Model file for the job. Use its own axes, mm. Give positions to 0.01 mm unless a question says otherwise; leave off trailing zeros. Order: outer loops, then holes, each group sorted by start corner. A loop starts at its lowest first (then second) coordinate and runs counter-clockwise, first axis right, second up. Notation, with made-up numbers: (6, 9) - (51, 9) arc R21 cw to (51, 14) - close; hole circle Ø11 at (8, 67). An arc over 180 degrees is marked (long way). Return JSON: item names as keys, results as strings. Group by question number.
from build123d import *

# Parameters (mm, degrees)
SKETCH1_W               = 180
SKETCH1_H               = 95
BOSS_EXTRUDE1_DEPTH     = 3.18
SKETCH2_W               = 3.18
SKETCH2_H               = 37.625
CUT_EXTRUDE1_DEPTH      = 1
CUT_EXTRUDE1_DEPTH_BACK = 4.18
SKETCH3_R               = 1.55
CUT_EXTRUDE2_DEPTH      = 1
CUT_EXTRUDE2_DEPTH_BACK = 4.18
CUT_EXTRUDE3_DEPTH      = 1
CUT_EXTRUDE3_DEPTH_BACK = 4.18
CUT_EXTRUDE4_DEPTH      = 1
CUT_EXTRUDE4_DEPTH_BACK = 4.18
CUT_EXTRUDE5_DEPTH      = 1
CUT_EXTRUDE5_DEPTH_BACK = 4.18
SKETCH8_W               = 58.994769075
SKETCH8_H               = 13
CUT_EXTRUDE6_DEPTH      = 1
CUT_EXTRUDE6_DEPTH_BACK = 4.18
SKETCH9_R               = 1.6
CUT_EXTRUDE7_DEPTH      = 1
CUT_EXTRUDE7_DEPTH_BACK = 4.18


with BuildPart() as part:
    # Sketch1 → Boss-Extrude1 (new body)
    with BuildSketch(Plane.XY):
        Rectangle(SKETCH1_W, SKETCH1_H)
    extrude(amount=BOSS_EXTRUDE1_DEPTH)

    # Sketch2 → Cut-Extrude1 (cut, two sides)
    with BuildSketch(Plane.XY.offset(3.18)) as cut_extrude1_sk:
        with Locations((88.41, 28.6875)):
            Rectangle(SKETCH2_W, SKETCH2_H)
        with Locations((88.41, -28.6875)):
            Rectangle(SKETCH2_W, SKETCH2_H)
    extrude(amount=CUT_EXTRUDE1_DEPTH, mode=Mode.SUBTRACT)
    extrude(cut_extrude1_sk.sketch, amount=-CUT_EXTRUDE1_DEPTH_BACK, mode=Mode.SUBTRACT)

    # Sketch3 → Cut-Extrude2 (cut, two sides)
    with BuildSketch(Plane.XY.offset(3.18)) as cut_extrude2_sk:
        with Locations((88, 0)):
            Circle(SKETCH3_R)
    extrude(amount=CUT_EXTRUDE2_DEPTH, mode=Mode.SUBTRACT)
    extrude(cut_extrude2_sk.sketch, amount=-CUT_EXTRUDE2_DEPTH_BACK, mode=Mode.SUBTRACT)

    # Sketch5 → Cut-Extrude3 (cut, two sides)
    with BuildSketch(Plane(origin=(0, 0, 0), x_dir=(-1, 0, 0), z_dir=(0, 0, -1))) as cut_extrude3_sk:
        Polygon((11.59, 47.5), (-8.41, 47.5), (-8.41, 44.32), (0.09, 44.32), (0.09, 40.32), (-1.91, 40.32), (-1.91, 37.5), (0.09, 37.5), (0.09, 34.5), (3.09, 34.5), (3.09, 37.5), (5.09, 37.5), (5.09, 40.32), (3.09, 40.32), (3.09, 44.32), (11.59, 44.32), align=None)
    extrude(amount=CUT_EXTRUDE3_DEPTH, mode=Mode.SUBTRACT)
    extrude(cut_extrude3_sk.sketch, amount=-CUT_EXTRUDE3_DEPTH_BACK, mode=Mode.SUBTRACT)

    # Sketch6 → Cut-Extrude4 (cut, two sides)
    with BuildSketch(Plane.XY.offset(3.18)) as cut_extrude4_sk:
        Polygon((-21.59, -47.5), (-1.59, -47.5), (-1.59, -44.32), (-10.09, -44.32), (-10.09, -40.32), (-8.09, -40.32), (-8.09, -37.5), (-10.09, -37.5), (-10.09, -34.5), (-13.09, -34.5), (-13.09, -37.5), (-15.09, -37.5), (-15.09, -40.32), (-13.09, -40.32), (-13.09, -44.32), (-21.59, -44.32), align=None)
    extrude(amount=CUT_EXTRUDE4_DEPTH, mode=Mode.SUBTRACT)
    extrude(cut_extrude4_sk.sketch, amount=-CUT_EXTRUDE4_DEPTH_BACK, mode=Mode.SUBTRACT)

    # Sketch7 → Cut-Extrude5 (cut, two sides)
    with BuildSketch(Plane.XY.offset(3.18)) as cut_extrude5_sk:
        Polygon((-90, 10), (-86.82, 10), (-86.82, 1.5), (-82.82, 1.5), (-82.82, 3.5), (-80, 3.5), (-80, 1.5), (-77, 1.5), (-77, -1.5), (-80, -1.5), (-80, -3.5), (-82.82, -3.5), (-82.82, -1.5), (-86.82, -1.5), (-86.82, -10), (-90, -10), align=None)
    extrude(amount=CUT_EXTRUDE5_DEPTH, mode=Mode.SUBTRACT)
    extrude(cut_extrude5_sk.sketch, amount=-CUT_EXTRUDE5_DEPTH_BACK, mode=Mode.SUBTRACT)

    # Sketch8 → Cut-Extrude6 (cut, two sides)
    with BuildSketch(Plane.XY.offset(3.18)) as cut_extrude6_sk:
        with Locations((-57.357372864, -23.3)):
            Rectangle(SKETCH8_W, SKETCH8_H)
    extrude(amount=CUT_EXTRUDE6_DEPTH, mode=Mode.SUBTRACT)
    extrude(cut_extrude6_sk.sketch, amount=-CUT_EXTRUDE6_DEPTH_BACK, mode=Mode.SUBTRACT)

    # Sketch9 → Cut-Extrude7 (cut, two sides)
    with BuildSketch(Plane.XY.offset(3.18)) as cut_extrude7_sk:
        with Locations((-4.59, -27.32)):
            Circle(SKETCH9_R)
        with Locations((43.41, -27.32)):
            Circle(SKETCH9_R)
    extrude(amount=CUT_EXTRUDE7_DEPTH, mode=Mode.SUBTRACT)
    extrude(cut_extrude7_sk.sketch, amount=-CUT_EXTRUDE7_DEPTH_BACK, mode=Mode.SUBTRACT)


solid = part.part
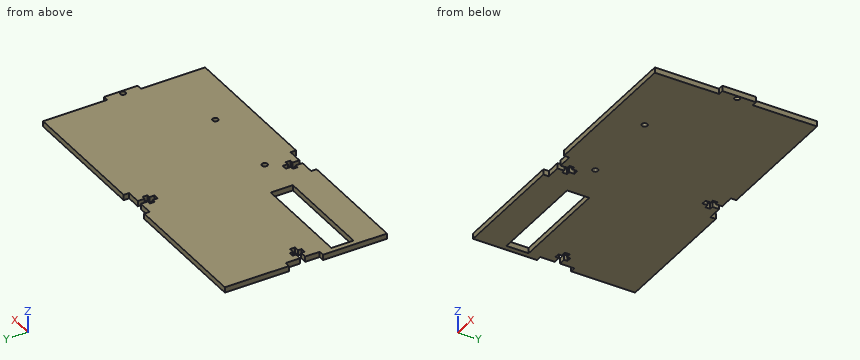
(1) Slice it at B-B (z = 1.95). State how many separate pieces and enclosed holes the cut face has, and give its area (3 significant figures).
(2) Drill centre lines: L1, parallel to Y at x = -4.59, z = 1.4; L2, parallel to X at y = -42, z = 1.3; L3, parallel to Y at x = 88, z = 1.2 (3 decimals). Where is each one in solid material? Low to high.
(3) Drop flat-ended pins along their axis: pin 1 Ø0.6 at (x, z) = (1, 1.5) entering from +Y; pin 2 Ø0.9 at (y, z) = (-36.5, 1.5) entering from +X; pin 3 Ø1 at (y, z) = (2, 1) entering from -X. Give the stop position or say it passes through.
(4) Slice it at A-A (x = -65). Give the cut face in (y, z), and give its area (3 significant figures).
Result set:
{
 "1": {"separate pieces": "1", "enclosed holes": "4", "area": "15,800 mm²"},
 "2": {"L1": "y = -44.32 to -28.92, -25.72 to 37.5, 40.32 to 44.32", "L2": "x = -90 to -13.09, -10.09 to 86.82", "L3": "y = -9.875 to -1.55, 1.55 to 9.875"},
 "3": {"pin 1": "stops at y = 44.32", "pin 2": "stops at x = 86.82", "pin 3": "stops at x = -86.82"},
 "4": {"outline": "(-47.5, 0) - (-29.8, 0) - (-29.8, 3.18) - (-47.5, 3.18) - close; (-16.8, 0) - (47.5, 0) - (47.5, 3.18) - (-16.8, 3.18) - close", "area": "261 mm²"}
}
